Geometry: final body of the model. Coordinates: model frame, mm. Give positions to 0.01 mm unless a question says otherwise; leave off trailing zeros. Write each loop counter-clockwise with the first axis right and the second up, starting at its lowest first coordinate (ties: lowest second). Pieces come first, ordered by that corner, then holes.
Q1. Cut plane A-A on y = 18.25. Return the cut outline in (x, z).
Q2. Line query: L1, parallel to Z at x = 119.5, y = 19.75; L2, parallel to Z at x = 60, y = 13; L3, parallel to Y at x = 99, z = -1. Output: solid intervals per line, ascending.
Q3. Draft query along Z for faces 1 (the face through (-2.1, 29.473, 0.648)), 2 (the face through (-2.1, 29.793, 0.655)). Return one class per face: pulls with the +Z half, pulls with the -Z half, needs draft (parallel to the pull), parting line crosses it, or undercut.
Q4. Pin query (flat end, axial travel): pin 1 (2.5 mm diameter, centred on x = -130, y = 27, fed in from +Z); pin 2 (1.8 mm diameter, centred on x = -130, y = 27, fed in from -Z); pin 3 (6 mm diameter, centred on x = 77, y = 15.5, fed in from +Z); pin 4 (4 mm diameter, centred on x = 37.5, z = -12, fed in from -Y). Return the tip coordinate at first contact, or that it passes through.
Q5. Cut plane C-C on x = -84.5. Return the cut outline in (y, z), plus the area to 3 significant figures.
Q6. Cut plane D-D on z = 3. Return the cut outline in (x, y).
Q7. Cut plane B-B on x = 0. Return the cut outline in (y, z).
Autodesk Inventor part; units mm, degrees
ref_plane "Work Plane1" through (0, 0, 29.8) normal (0, 0, 1) x (1, 0, 0)
ref_plane "YZ Plane" through (0, 0, 0) normal (1, 0, 0) x (0, 1, 0)
ref_plane "XZ Plane" through (0, 0, 0) normal (0, 1, 0) x (-1, 0, 0)
sketch "Sketch1" plane through (0, 0, 0) normal (1, 0, 0) x (0, 1, 0)
  arc A0 (0, -29.8) -> (0, 29.8) centre (0, 0) ccw
  arc A1 (0, -29.48) -> (0, 29.48) centre (0, 0) ccw
  line L0 (0, -29.8) -> (0, -29.48)
  line L1 (0, 29.48) -> (0, 29.8)
  dimension "d0" = 29.8
  dimension "d1" = 59.6
  dimension "d4" = 29.48
extrude "Extrusion1" add sketch "Sketch1" along normal mid plane 300
sketch "Sketch2" plane through (0, 0, 0) normal (0, 0, 1) x (1, 0, 0)
  line L0 (-150, 0) -> (150, 0)
  line L1 (-150, 0) -> (150, 0)
  line L2 (150, 0) -> (150, 0)
  line L3 (150, 0) -> (-150, 0)
  line L4 (-150, 0) -> (-150, 0)
  point P0 (0, 0)
  point P1 (0, 10)
  point P2 (-134.6305, 7.2182)
  dimension "d7" = 10
hole "Hole1" at (0, 10, 0) direction (0, 0, -1) diameter 5.4 end through all both
ref_plane "Work Plane1" through (0, 0, 29.8) normal (0, 0, 1) x (1, 0, 0)
sketch "Sketch3" plane through (0, 0, 29.8) normal (0, 0, 1) x (1, 0, 0)
  line L0 (-150, 29.8) -> (-150, 0)
  line L1 (-150, 0) -> (150, 0)
  line L2 (150, 0) -> (150, 29.8)
  point P0 (0, 0)
  point P1 (-130, 27)
  point P2 (130, 27)
  dimension "d16" = 20
  dimension "d17" = 27
  dimension "d19" = 260
hole "Hole2" at (-130, 27, 29.8) at (130, 27, 29.8) direction (0, 0, -1) diameter 2 end through all
properties part number "tubo PVC"
Data:
1. outline: (-150, -23.56) - (150, -23.56) - (150, -23.15) - (-150, -23.15) - close; (-150, 23.15) - (150, 23.15) - (150, 23.56) - (-150, 23.56) - close
2. L1: z = -22.32 to -21.89, 21.89 to 22.32
2. L2: z = -26.81 to -26.46, 26.46 to 26.81
2. L3: y = 29.46 to 29.78
3. face 1: undercut
3. face 2: parting line crosses it
4. pin 1: stops at z = 15
4. pin 2: passes through
4. pin 3: stops at z = 27.05
4. pin 4: stops at y = 25.94
5. outline: (0, -29.8) arc R29.8 ccw to (0, 29.8) - (0, 29.48) arc R29.48 cw to (0, -29.48) - close
5. area: 29.8 mm2
6. outline: (-150, 29.33) - (150, 29.33) - (150, 29.65) - (-150, 29.65) - close
7. outline: (0, -29.8) arc R29.8 ccw to (7.3, -28.89) - (7.3, -28.56) arc R29.48 cw to (0, -29.48) - close; (0, 29.48) arc R29.48 cw to (7.3, 28.56) - (7.3, 28.89) arc R29.8 ccw to (0, 29.8) - close; (12.7, -26.96) arc R29.8 ccw to (12.7, 26.96) - (12.7, 26.6) arc R29.48 cw to (12.7, -26.6) - close
